from build123d import *

# Parameters (mm, degrees)
SKETCH1_W                  = 310
SKETCH1_H                  = 130
BOSS_EXTRUDE1_DEPTH        = 3
FILLET1_R                  = 4
F_5_3_5_3_DIAMETER_HOLE1_D = 5.3
SKETCH6_W                  = 180
SKETCH6_H                  = 45
CUT_EXTRUDE1_DEPTH         = 4
FILLET2_R                  = 5
M5X0_8_TAPPED_HOLE1_D      = 4.2
CUT_EXTRUDE2_DEPTH         = 4


with BuildPart() as part:
    # Sketch1 → Boss-Extrude1 (new body)
    with BuildSketch(Plane(origin=(0, 0, 0), x_dir=(1, 0, 0), z_dir=(0, 1, 0))):
        Rectangle(SKETCH1_W, SKETCH1_H)
    extrude(amount=BOSS_EXTRUDE1_DEPTH)

    # Fillet1
    fillet1_edges = [part.edges().sort_by_distance(p)[0] for p in [
        (155, 1.5, 65),
        (-155, 1.5, 65),
        (-155, 1.5, -65),
        (155, 1.5, -65),
    ]]
    fillet(fillet1_edges, radius=FILLET1_R)

    # Ø5.3 (5.3) Diameter Hole1 (through all)
    with Locations(Plane(origin=(0, 3, 0), x_dir=(1, 0, 0), z_dir=(0, 1, 0))):
        with Locations((125, 55), (-125, -55), (-125, 55), (125, -55)):
            Hole(F_5_3_5_3_DIAMETER_HOLE1_D / 2)

    # Sketch6 → Cut-Extrude1 (cut, through all)
    with BuildSketch(Plane(origin=(0, 3, 0), x_dir=(1, 0, 0), z_dir=(0, 1, 0))):
        with Locations((-35, -5)):
            Rectangle(SKETCH6_W, SKETCH6_H)
    extrude(amount=-CUT_EXTRUDE1_DEPTH, mode=Mode.SUBTRACT)

    # Fillet2
    fillet2_edges = [part.edges().sort_by_distance(p)[0] for p in [
        (55, 1.5, -17.5),
        (55, 1.5, 27.5),
        (-125, 1.5, 27.5),
        (-125, 1.5, -17.5),
    ]]
    fillet(fillet2_edges, radius=FILLET2_R)

    # M5x0.8 Tapped Hole1 (through all)
    with Locations(Plane(origin=(0, 3, 0), x_dir=(1, 0, 0), z_dir=(0, 1, 0))):
        with Locations((67, -3.5), (-137, -21.5), (-137, -3.5), (67, -21.5)):
            Hole(M5X0_8_TAPPED_HOLE1_D / 2)

    # Sketch9 → Cut-Extrude2 (cut, through all)
    with BuildSketch(Plane(origin=(0, 3, 0), x_dir=(1, 0, 0), z_dir=(0, 1, 0))):
        with BuildLine():
            Line((-127.65, 53.5), (-127.65, 56.5))
            ThreePointArc((-127.65, 56.5), (-125, 59.15), (-122.35, 56.5))
            Line((-122.35, 56.5), (-122.35, 53.5))
            ThreePointArc((-122.35, 53.5), (-125, 50.85), (-127.65, 53.5))
        make_face()
        with BuildLine():
            Line((122.35, 53.5), (122.35, 56.5))
            ThreePointArc((122.35, 56.5), (125, 59.15), (127.65, 56.5))
            Line((127.65, 56.5), (127.65, 53.5))
            ThreePointArc((127.65, 53.5), (125, 50.85), (122.35, 53.5))
        make_face()
    extrude(amount=-CUT_EXTRUDE2_DEPTH, mode=Mode.SUBTRACT)


solid = part.part
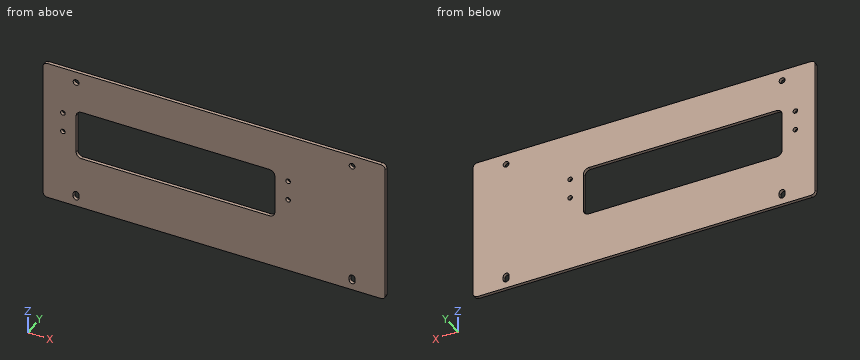
Geometry check sheet. Reference: the model listing, model coordinates, mm. Round coordinates to 2 decimals unless told otherwise and drop trailing zeros. Order: outer loops, then holes, each group sorted by start corner. A loop starts at its lowest first (then second) coordinate and runs counter-clockwise, first axis right, second up. Notation, with made-up numbers: (4, 33.5) - (55, 33.5) arc R23 cw to (55, 46.5) - close; hole circle Ø7 at (12, 1.25). An arc over 180 degrees is marked (long way). One line per question, with ' | ' between items. Start each with the question number.
(1) Sectioned sample at B-B on z = 13.5. Record the cut outline in (x, y).
(2) Depth check by flat-ended pin: pin 1 Ø3 at (x, z) = (-125, 55) entering from +Y. Enter the tip coordinate at first touch or a pass-through.
(3) Sectioned sample at C-C on y = 2.45. Count the separate pieces of the cut face and the enclosed holes in it, and give its area (3 significant figures).
(4) Thickness scan on L1, parallel to X at y = 1.45, z = 55; L2, parallel to X at y = 2.1, z = 18.5; L3, parallel to X at y = 1.8, z = 21.5. Record the ranges inside material, lowest first. Write a range as [from, to].
(5) Sectioned sample at A-A on x = 7. Record the cut outline in (y, z).
Conclusion:
1) outline: (-155, 0) - (-125, 0) - (-125, 3) - (-155, 3) - close; (55, 0) - (155, 0) - (155, 3) - (55, 3) - close
2) pin 1: passes through
3) separate pieces: 1 | enclosed holes: 9 | area: 32,000 mm2
4) L1: x = [-155, -127.65], [-122.35, 122.35], [127.65, 155] | L2: x = [-155, -125], [55, 155] | L3: x = [-155, -139.1], [-134.9, -125], [55, 64.9], [69.1, 155]
5) outline: (0, -65) - (3, -65) - (3, -17.5) - (0, -17.5) - close; (0, 27.5) - (3, 27.5) - (3, 65) - (0, 65) - close
